```python
from build123d import *

# Parameters (mm, degrees)
F0_R     = 2.5
F1_DEPTH = 2
F2_R     = 0.99999


# Not quite as in the source:
# - a fillet or chamfer is up to 0.001 mm smaller than in the source, because OpenCascade refuses the exact size


with BuildPart() as f1:
    # F0 (on Top) → F1 (new body)
    with BuildSketch(Plane.XY):
        Polygon((-7.5, 101.8), (-7.5, -4.85), (7.5, -4.85), (7.5, 3.15), (25.5, 3.15), (25.5, -4.85), (35.5, -4.85), (35.5, 3.15), (39.5, 3.15), (39.5, -9.35), (50.65, -9.35), (50.65, 0), (52.65, 0), (52.65, -9.35), (90.8, -9.35), (90.8, 3.15), (160.15, 3.15), (160.15, 101.8), align=None)
        Circle(F0_R, mode=Mode.SUBTRACT)
        with Locations((0, 85.4)):
            Circle(F0_R, mode=Mode.SUBTRACT)
    extrude(amount=F1_DEPTH)

    # F2 (radius 1 in the source; OpenCascade refuses exactly that, so slightly less here)
    f2_edges = [f1.edges().sort_by_distance(p)[0] for p in [
        (-7.5, -4.85, 1),
        (7.5, -4.85, 1),
        (25.5, 3.15, 1),
        (25.5, -4.85, 1),
        (35.5, -4.85, 1),
        (39.5, 3.15, 1),
        (39.5, -9.35, 1),
        (50.65, -9.35, 1),
        (52.65, 0, 1),
        (52.65, -9.35, 1),
        (90.8, -9.35, 1),
        (-7.5, 101.8, 1),
        (160.15, 101.8, 1),
        (160.15, 3.15, 1),
        (90.8, 3.15, 1),
        (35.5, 3.15, 1),
        (7.5, 3.15, 1),
        (50.65, 0, 1),
    ]]
    fillet(f2_edges, radius=F2_R)


solid = f1.part
```
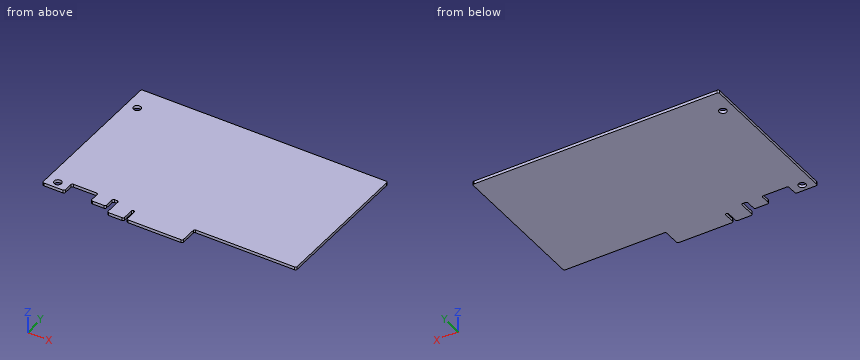
CAD build for the part. Positions are in the model's coordinates, mm. Round coordinates to 2 decimals unless told otherwise and drop trailing zeros. Write each loop counter-clockwise with the first axis right and the second up, starting at its lowest first coordinate (ties: lowest second). Pieces come first, ordered by that corner, then holes. Notation, with made-up numbers: M 58,-17.5 L 90,-17.5 A14 cw 90,-4.5 Z; hole C 39,-16.5 d5. An arc over 180 degrees is marked long. One line per question, with ' | ' between items.
1. Cut at B-B on z = 0.35. Count the separate pieces of the cut face and the enclosed holes in it, and give its area (3 significant figures).
Working result:
separate pieces: 1 | enclosed holes: 2 | area: 17,300 mm2
2. Cut at C-C on x = 134. Write the cut outline in (y, z).
Working result:
outline: M 3.15,0 L 101.8,0 L 101.8,2 L 3.15,2 Z
3. Pin check, flat tips, straight feed: pin 1 Ø6 at (x, y) = (0, 85.4) entering from +Z; pin 2 Ø0.6 at (x, z) = (32.5, 1) entering from -Y; pin 3 Ø1 at (y, z) = (-6, 0.5) entering from -X; pin 4 Ø0.6 at (y, z) = (-2.5, 1.5) entering from +X. Stop position of each tip, or through.
Working result:
pin 1: z = 2 | pin 2: y = -4.85 | pin 3: x = 39.5 | pin 4: x = 90.8
4. Probe L1, parallel to Y at x = 0, z = 0.95; L2, parallel to X at y = -0.5, z = 0.6; L3, parallel to Y at x = 146, z = 0.9. List the from-to ranges inside material, lowest first. Write a range as from..to.
Working result:
L1: -4.85..-2.5, 2.5..82.9, 87.9..101.8 | L2: -7.5..-2.45, 2.45..7.5, 25.5..35.5, 39.5..50.78, 52.52..90.8 | L3: 3.15..101.8
5. Cut at A-A on x = 0. Write the cut outline in (y, z).
Working result:
outline: M -4.85,0 L -2.5,0 L -2.5,2 L -4.85,2 Z; M 2.5,0 L 82.9,0 L 82.9,2 L 2.5,2 Z; M 87.9,0 L 101.8,0 L 101.8,2 L 87.9,2 Z
